For this review, take the finished solid that the model builds, in its own axes (mm). A direction names the side the tool comes from. Coordinates: 2 decimals unless noted, no trailing zeros. Write each loop counter-clockwise with the first axis right and the second up, starting at its lowest first coordinate (ties: lowest second). Pieces come first, ordered by that corner, then holes.
1) Mouldability with a two-part tool opening along Y and no side actions: class faces 4 (the face through (0, 0, 11)), 5 (the face through (-10, 0, 6)), 6 (the face through (0, 0, 1)), 7 (the face through (-2.4, 4, 5.9)) as pulls with the +Y half, pulls with the -Y half, needs draft (parallel to the pull), parting line crosses it, or undercut.
2) We need section A-A on z = 11.25. Write out the cut boundary in (x, y).
3) To check wall thickness, follow line 1 along Y through (x, z) = (9.25, 11.25); line 2 along X through (y, z) = (-1, 5); line 3 along Z through (x, y) = (8.5, 1). State the ranges of each line that lie inside material, in increasing order.
4) For faces 1 (the face through (0.1, 2, 11.5)), 2 (the face through (0.1, 2, 0.5)), 3 (the face through (0, -3, 0)), list the 3-axis set-ups (+Z, -Z, +X, -X, +Y, -Y) from which the entire face can be reached by the end or side of a thin tool; tool diameter is ignored.
5) Insertion check: P1, Ø2, axis at x = 2.5, y = 0.5, coming from the +Z side. The pin has a flat end and moves straight along its axis. Give the tip position at first contact, or say it passes through.
6) We need section B-B on y = -1. Write out the cut boundary in (x, z).
7) We need section D-D on y = 3.75. Write out the cut boundary in (x, z), then the cut area to 3 significant figures.
8) We need section C-C on x = -3.5. Write out the cut boundary in (y, z).
from build123d import *

# Parameters (mm, degrees)
SKETCH_1_W          = 20
SKETCH_1_H          = 8
EXTRUDE_1_DEPTH     = 12
SKETCH_2_W          = 1
SKETCH_2_H          = 4
CUT_EXTRUDE_3_DEPTH = 21
CUT_EXTRUDE_4_DEPTH = 9


with BuildPart() as part:
    # 草图1 → 凸台-拉伸1 (new body)
    with BuildSketch(Plane.XY):
        Rectangle(SKETCH_1_W, SKETCH_1_H)
    extrude(amount=EXTRUDE_1_DEPTH)

    # 草图2 → 切除-拉伸3 (cut, through all)
    with BuildSketch(Plane(origin=(10, 0, 0), x_dir=(0, 0, -1), z_dir=(1, 0, 0))):
        with Locations((-0.5, 0)):
            Rectangle(SKETCH_2_W, SKETCH_2_H)
        with Locations((-11.5, 0)):
            Rectangle(SKETCH_2_W, SKETCH_2_H)
    extrude(amount=-CUT_EXTRUDE_3_DEPTH, mode=Mode.SUBTRACT)

    # 草图3 → 切除-拉伸4 (cut, through all)
    with BuildSketch(Plane(origin=(0, 4, 0), x_dir=(1, 0, 0), z_dir=(0, 1, 0))):
        with BuildLine():
            ThreePointArc((2, -6), (1.414213562, -4.585786438), (0, -4))
            Line((0, -4), (0, -8))
            ThreePointArc((0, -8), (1.414213562, -7.414213562), (2, -6))
        make_face()
        with BuildLine():
            Line((0, -8), (0, -4))
            ThreePointArc((0, -4), (-2, -6), (0, -8))
        make_face()
    extrude(amount=-CUT_EXTRUDE_4_DEPTH, mode=Mode.SUBTRACT)


solid = part.part
Result:
1. face 4: undercut
1. face 5: needs draft
1. face 6: undercut
1. face 7: pulls with the +Y half
2. outline: (-10, -4) - (10, -4) - (10, -2) - (-10, -2) - close; (-10, 2) - (10, 2) - (10, 4) - (-10, 4) - close
3. line 1: y = -4 to -2, 2 to 4
3. line 2: x = -10 to -1.73, 1.73 to 10
3. line 3: z = 1 to 11
4. face 1: +Z, +X, -X
4. face 2: -Z, +X, -X
4. face 3: -Z, +X, -X, +Y, -Y
5. P1: stops at z = 11
6. outline: (-10, 1) - (10, 1) - (10, 11) - (-10, 11) - close; hole circle Ø4 at (0, 6)
7. outline: (-10, 0) - (10, 0) - (10, 12) - (-10, 12) - close; hole circle Ø4 at (0, 6)
7. area: 227 mm2
8. outline: (-4, 0) - (-2, 0) - (-2, 1) - (2, 1) - (2, 0) - (4, 0) - (4, 12) - (2, 12) - (2, 11) - (-2, 11) - (-2, 12) - (-4, 12) - close
